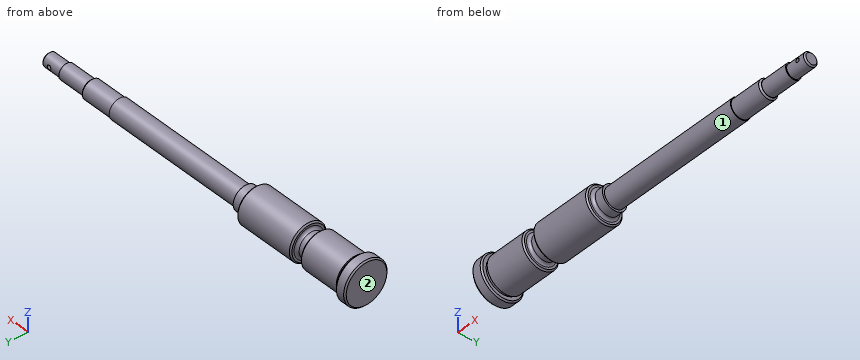
```python
from build123d import *

# Parameters (mm, degrees)
CHAMFER_1_SIZE = 1
FILLET_1_R     = 2
FILLET_2_R     = 2


# Read off the part's stored shape, not the designer's step: M14 机械螺纹 螺柱1
with BuildPart() as part:
    # 草图1 → 旋转1 (revolve)
    with BuildSketch(Plane.XY, mode=Mode.PRIVATE) as revolve_1_sk:
        Polygon((0, 0), (0, 16), (8, 16), (8, 12.5), (10, 12.5), (10, 13.5), (40, 13.5), (40, 9), (48, 9), (48, 13.5), (93, 13.5), (93, 9), (101, 9), (101, 7.5), (230, 7.5), (230, 5.75), (250, 5.75), (250, 5), (265, 5), (265, 0), align=None)
    revolve(revolve_1_sk.sketch.rotate(Axis((0, 0, 0), (1, 0, 0)), 90), axis=Axis((0, 0, 0), (1, 0, 0)))

    # M14 机械螺纹 螺柱1 outline → M14 机械螺纹 螺柱1 (revolve, cut)
    with BuildSketch(Plane.YX):
        Polygon((7.5, 230), (5.9175, 230), (7, 228.9175), (7, 206), (7.5, 206), align=None)
    revolve(axis=Axis((0, 0, 0), (1, 0, 0)), mode=Mode.SUBTRACT)

    # 草图3 → 切除-旋转1 (revolve, cut)
    with BuildSketch(Plane.XY, mode=Mode.PRIVATE) as cut_revolve_1_sk:
        Polygon((259, -5.697872022), (260.4, -5.697872022), (260.5, 5.677594139), (259, 5.677594139), align=None)
    revolve(cut_revolve_1_sk.sketch.rotate(Axis((259, -22.643842163, 0), (0, 1, 0)), 131.522767303), axis=Axis((259, -22.643842163, 0), (0, 1, 0)), mode=Mode.SUBTRACT)

    # 倒角1
    chamfer_1_edges = [part.edges().sort_by_distance(p)[0] for p in [
        (265, 0, -5),
        (93, 0, -13.5),
        (48, 0, -13.5),
        (40, 0, -13.5),
        (8, 0, -16),
        (0, 0, -16),
    ]]
    chamfer(chamfer_1_edges, length=CHAMFER_1_SIZE)

    # 圆角1
    fillet_1_edges = [part.edges().sort_by_distance(p)[0] for p in [
        (48, 0, -9),
        (40, 0, -9),
    ]]
    fillet(fillet_1_edges, radius=FILLET_1_R)

    # 圆角2
    fillet_2_edges = [part.edges().sort_by_distance(p)[0] for p in [
        (93, 0, -9),
    ]]
    fillet(fillet_2_edges, radius=FILLET_2_R)


solid = part.part
```
The model under review builds one solid part; all positions refer to its coordinate system, in mm. Face numbers are marked on the shaded views. Round coordinates to 2 decimals unless told otherwise and drop trailing zeros. Loops run counter-clockwise (first coordinate to the right, second up) from the corner with the lowest first, then second, coordinate; pieces in that order, holes last. Notation, with made-up numbers: (21, 83) -> (35, 83) arc R23 cw to (35, 113) -> close; hole circle Ø2 at (52, -8.75). An arc over 180 degrees is marked (long way). Answer as a JSON object with one key per item and string values. Group by question number.
1) We need section A-A on x = 34. Write out the cut boundary in (y, z).
2) For line 1 (X direction, y = -2.5, z = -11.5); line 2 (X direction, y = 4, z = -12); line 3 (Y direction, x = 48.5, z = -7), list the stretches that pass through material, from the lowest coordinate up. Write a range as [from, to].
3) We need section B-B on x = 136. Write out the cut boundary in (y, z).
4) Mouldability with a two-part tool opening along X and no side actions: class the marked faces 1 and 2 as released by +X, released by -X, zero draft, split by the parting line, or undercut.
5) For pin 1 Ø5 at (x, z) = (149, 9) entering from +Y; pin 2 Ø4 at (x, z) = (118.5, 4) entering from +Y; pin 3 Ø3 at (x, y) = (68, -6.5) entering from -Z; pin 4 Ø6 at (x, z) = (151.5, -11.5) entering from -Y, all flat-tipped, find the tip position at first contact; note any pin that passes through.
Result set:
{
 "1": {"outline": "circle Ø27 at (0, 0)"},
 "2": {"line 1": "[0, 40], [48, 93]", "line 2": "[0, 8], [10, 39.85], [48.15, 92.85]", "line 3": "[-10.95, 10.95]"},
 "3": {"outline": "circle Ø15 at (0, 0)"},
 "4": {"face 1": "zero draft", "face 2": "released by -X"},
 "5": {"pin 1": "y = 3.74", "pin 2": "y = 7.23", "pin 3": "z = -12.54", "pin 4": "through"}
}
